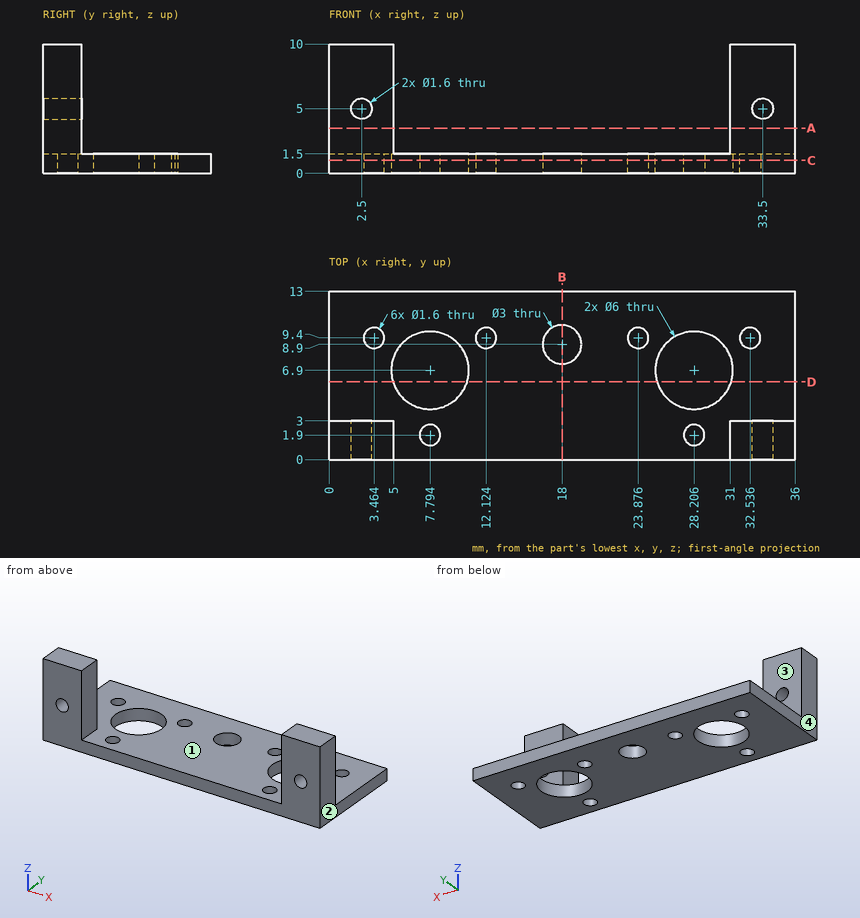
Part print with two shaded views. Sizes in mm from the minimum x, y, z corner. Round coordinates to 2 decimals unless told otherwise and drop trailing zeros. Write each loop counter-clockwise with the first axis right and the second up, starting at its lowest first coordinate (ties: lowest second). Pieces come first, ordered by that corner, then holes. Notation, with made-up numbers: (83.25, -4.5) -> (114.25, -4.5) arc R22 ccw to (114.25, 34.5) -> close; hole circle Ø4 at (17.5, -27.75). An arc over 180 degrees is marked (long way). Put each result on its own line as item: value.
Item 1: Slice it at C-C, the plane z = 1. Count the separate pieces of the cut face and the enclosed holes in it, plus the area to 3 significant figures.
Here are the results:
separate pieces: 1
enclosed holes: 9
area: 392 mm^2
Item 2: Two-plate mould, pull along X, no slides. Class the marked faces 1, 2, 3 and 4: pulls with the +X half, pulls with the -X half, needs draft (parallel to the pull), parting line crosses it, or undercut.
Here are the results:
face 1: undercut
face 2: pulls with the +X half
face 3: needs draft
face 4: pulls with the -X half
Item 3: Slice it at D-D, the plane y = 6. Give the cut face in (x, z).
Here are the results:
outline: (0, 0) -> (4.93, 0) -> (4.93, 1.5) -> (0, 1.5) -> close; (10.66, 0) -> (25.34, 0) -> (25.34, 1.5) -> (10.66, 1.5) -> close; (31.07, 0) -> (36, 0) -> (36, 1.5) -> (31.07, 1.5) -> close
Item 4: Slice it at B-B, the plane x = 18. Give the cut face in (y, z), plus the area to 3 significant figures.
Here are the results:
outline: (0, 0) -> (7.4, 0) -> (7.4, 1.5) -> (0, 1.5) -> close; (10.4, 0) -> (13, 0) -> (13, 1.5) -> (10.4, 1.5) -> close
area: 15.0 mm^2
Item 5: Wall check: probe 1 along X at (y, z) = (6.9, 0.85); probe 2 along X at (y, z) = (1.4, 5); probe 3 along X at (y, z) = (1.9, 1.2). Give the ranges that are in metal, low to high. Write a range as from..to.
Here are the results:
probe 1: x = 0..4.79, 10.79..25.21, 31.21..36
probe 2: x = 0..1.7, 3.3..5, 31..32.7, 34.3..36
probe 3: x = 0..6.99, 8.59..27.41, 29.01..36
Item 6: Slice it at A-A, the plane z = 3.5. Give the cut face in (x, y), plus the area to 3 significant figures.
Here are the results:
outline: (0, 0) -> (5, 0) -> (5, 3) -> (0, 3) -> close; (31, 0) -> (36, 0) -> (36, 3) -> (31, 3) -> close
area: 30.0 mm^2
Item 7: Flat gauge pins, fed straight in: P1, Ø2, axis at x = 2.5, z = 5, coming from the +Y side; P2, Ø6, axis at y = 4, z = 7.5, coming from the +X side; P3, Ø4, axis at x = 18, y = 8.9, coming from the +Z side. Where does each tip first touch, or does it go through?
Here are the results:
P1: stops at y = 3
P2: stops at x = 36
P3: stops at z = 1.5
